```python
from build123d import *

# Parameters (mm, degrees)
F0_W     = 82.55
F0_H     = 82.55
F1_DEPTH = 152.4
F2_R     = 6.35
F3_R     = 6.35
F4_DEPTH = 28.575
F5_R     = 3.175
F6_DEPTH = 25.4


with BuildPart() as f1:
    # F0 (on Front) → F1 (new body)
    with BuildSketch(Plane.XZ):
        with Locations((41.275, 41.275)):
            Rectangle(F0_W, F0_H)
    extrude(amount=F1_DEPTH)

    # F2
    f2_edges = [f1.edges().sort_by_distance(p)[0] for p in [
        (0, -76.2, 82.55),
        (0, -76.2, 0),
        (82.55, -76.2, 82.55),
        (82.55, -76.2, 0),
    ]]
    fillet(f2_edges, radius=F2_R)

    # F3 (on face) → F4 (join)
    with BuildSketch(Plane.XZ.offset(152.4)):
        with Locations((41.275, 41.275)):
            Circle(F3_R)
    extrude(amount=F4_DEPTH)

    # F5 (on face) → F6 (cut)
    with BuildSketch(Plane.XZ.offset(152.4)):
        with Locations((6.35, 76.2)):
            Circle(F5_R)
        with Locations((6.35, 6.35)):
            Circle(F5_R)
        with Locations((76.2, 76.2)):
            Circle(F5_R)
        with Locations((76.2, 6.35)):
            Circle(F5_R)
    extrude(amount=-F6_DEPTH, mode=Mode.SUBTRACT)


solid = f1.part
```
Design review of the part built by this model. Coordinates are the model's own, in mm. A direction names the side the tool comes from. Round coordinates to 2 decimals unless told otherwise and drop trailing zeros. Order: outer loops, then holes, each group sorted by start corner. A loop starts at its lowest first (then second) coordinate and runs counter-clockwise, first axis right, second up. Notation, with made-up numbers: M 87.25,-34 L 114.25,-34 A19 cw 114.25,-6 Z; hole C 58.5,11.5 d7. An arc over 180 degrees is marked long. Put each result on its own line as item: value.
Q1. Draft analysis for pull direction X (two halves, no side actions). For faces 3 (the face through (76, -127, 76)), 4 (the face through (1.81, -77.27, 80.64)), 5 (the face through (41, 0, 42)), state which applies: released by +X, released by -X, zero draft, split by the parting line, or undercut.
Reported:
face 3: undercut
face 4: released by -X
face 5: zero draft
Q2. Machinability: for faces 1 (the face through (41, -180.975, 41)), 2 (the face through (4.01, -139.878, 78.346)), which of the approach directions +Z, -Z, +X, -X, +Y, -Y give a long, thin tool a straight path to every point of the face, cutting with its end or side? Answer none if there is none.
Reported:
face 1: +Z, -Z, +X, -X, -Y
face 2: -Y
Q3. To check wall thickness, follow line 1 (X direction, y = -132, z = 76); line 2 (Z direction, x = 6, y = -141). State the ranges of each line that lie inside material, in increasing order.
Reported:
line 1: 0 to 3.18, 9.52 to 73.03, 79.37 to 82.55
line 2: 0.01 to 3.19, 9.51 to 73.04, 79.36 to 82.54
Q4. Consider section B-B (x = 52). State the section outline as (y, z) points, and give its area (3 significant figures).
Reported:
outline: M -152.4,0 L 0,0 L 0,82.55 L -152.4,82.55 Z
area: 12,600 mm²
Q5. Consider section C-C (z = 54). State the section outline as (x, y) points.
Reported:
outline: M 0,-152.4 L 82.55,-152.4 L 82.55,0 L 0,0 Z
Q6. Insertion check: pin 1 Ø5 at (x, z) = (76.2, 76.2) entering from -Y; pin 2 Ø12 at (x, z) = (73, 48.5) entering from -Y. Each pin has a flat end and moves straight along its axis. Give the tip position at first contact, or say it passes through.
Reported:
pin 1: y = -127
pin 2: y = -152.4
Q7. Consider section A-A (y = -130.5). State the section outline as (x, z) points (3 decimals).
Reported:
outline: M 0,6.35 A6.35 ccw 6.35,0 L 76.2,0 A6.35 ccw 82.55,6.35 L 82.55,76.2 A6.35 ccw 76.2,82.55 L 6.35,82.55 A6.35 ccw 0,76.2 Z; hole C 6.35,6.35 d6.35; hole C 6.35,76.2 d6.35; hole C 76.2,6.35 d6.35; hole C 76.2,76.2 d6.35
